from build123d import *
from OCP.BRepFilletAPI import BRepFilletAPI_MakeChamfer

# Parameters (mm, degrees)
SKETCH1_R           = 4.765
BOSS_EXTRUDE1_DEPTH = 9.5
CHAMFER1_SIZE       = 2.54
CHAMFER1_SIZE2      = 7.62
CHAMFER2_SIZE       = 7.62
CHAMFER2_SIZE2      = 2.45
CUT_EXTRUDE1_DEPTH  = 17.5
SKETCH3_W           = 9.53
SKETCH3_H           = 9.53
CUT_EXTRUDE2_DEPTH  = 17.5
SKETCH4_R           = 1.59
CUT_EXTRUDE3_DEPTH  = 17.5


with BuildPart() as part:
    # Sketch1 → Boss-Extrude1 (new, symmetric)
    with BuildSketch(Plane(origin=(0, 0, 0), x_dir=(0, 0, -1), z_dir=(1, 0, 0))):
        with BuildLine():
            Line((0, 9.765), (-22.225, 9.765))
            Line((-22.225, 9.765), (-22.225, 4.765))
            Line((-22.225, 4.765), (-9.705896356, -1.072753903))
            ThreePointArc((-9.705896356, -1.072753903), (-5.873116096, -7.801392973), (1.653013564, -9.624072483))
            Line((1.653013564, -9.624072483), (28.575, -5))
            Line((28.575, -5), (28.575, 0))
            Line((28.575, 0), (9.765, 0))
            ThreePointArc((9.765, 0), (6.904897718, 6.904897718), (0, 9.765))
        make_face()
        Circle(SKETCH1_R, mode=Mode.SUBTRACT)
    extrude(amount=BOSS_EXTRUDE1_DEPTH, both=True)

    # Chamfer1: one chamfer whose edges measure the first distance from different faces: ONE call of the kernel's chamfer builder (chamfer() names one face for all edges)
    chamfer1_edges_1 = [part.edges().sort_by_distance(p)[0] for p in [
        (9.5, 7.265, 22.225),
    ]]
    chamfer1_side_1 = [part.faces().sort_by_distance(p)[0] for p in [
        (0, 7.265, 22.225),
    ]]
    chamfer1_edges_2 = [part.edges().sort_by_distance(p)[0] for p in [
        (9.5, -2.5, -28.575),
    ]]
    chamfer1_side_2 = [part.faces().sort_by_distance(p)[0] for p in [
        (0, -2.5, -28.575),
    ]]
    chamfer1 = BRepFilletAPI_MakeChamfer(part.part.solid().wrapped)
    for e in chamfer1_edges_1:
        chamfer1.Add(CHAMFER1_SIZE, CHAMFER1_SIZE2, e.wrapped, chamfer1_side_1[0].wrapped)  # the first distance lies on this face
    for e in chamfer1_edges_2:
        chamfer1.Add(CHAMFER1_SIZE, CHAMFER1_SIZE2, e.wrapped, chamfer1_side_2[0].wrapped)  # the first distance lies on this face
    add(Compound.cast(chamfer1.Shape()), mode=Mode.REPLACE)

    # Chamfer2
    chamfer2_edges = [part.edges().sort_by_distance(p)[0] for p in [
        (-9.5, 7.265, 22.225),
        (-9.5, -2.5, -28.575),
    ]]
    chamfer2_side = [part.faces().sort_by_distance(p)[0] for p in [
        (-9.5, 9.220751812, 11.1125),
    ]]
    chamfer(chamfer2_edges, length=CHAMFER2_SIZE, length2=CHAMFER2_SIZE2, reference=chamfer2_side[0])

    # Sketch2 → Cut-Extrude1 (cut, symmetric)
    with BuildSketch(Plane(origin=(0, 0, 0), x_dir=(1, 0, 0), z_dir=(0, 1, 0))):
        with BuildLine():
            Line((5.08, 6.35), (5.08, -3.81))
            ThreePointArc((5.08, -3.81), (0, -8.89), (-5.08, -3.81))
            Line((-5.08, -3.81), (-5.08, 6.35))
            ThreePointArc((-5.08, 6.35), (0, 11.43), (5.08, 6.35))
        make_face()
    extrude(amount=CUT_EXTRUDE1_DEPTH, both=True, mode=Mode.SUBTRACT)

    # Sketch3 → Cut-Extrude2 (cut, symmetric)
    with BuildSketch(Plane(origin=(0, 0, 0), x_dir=(1, 0, 0), z_dir=(0, 1, 0))):
        with Locations((0, 23.81)):
            Rectangle(SKETCH3_W, SKETCH3_H)
        with Locations((0, -17.46)):
            Rectangle(SKETCH3_W, SKETCH3_H)
    extrude(amount=CUT_EXTRUDE2_DEPTH, both=True, mode=Mode.SUBTRACT)

    # Sketch4 → Cut-Extrude3 (cut, symmetric)
    with BuildSketch(Plane(origin=(0, 0, 0), x_dir=(0, 0, -1), z_dir=(1, 0, 0))):
        with Locations((-19.685, 7.225)):
            Circle(SKETCH4_R)
        with Locations((26.035, -2.5)):
            Circle(SKETCH4_R)
    extrude(amount=CUT_EXTRUDE3_DEPTH, both=True, mode=Mode.SUBTRACT)


solid = part.part
Part model, mm, in its own coordinate system. A direction names the side the tool comes from. Coordinates: 2 decimals unless noted, no trailing zeros. Loops run counter-clockwise (first coordinate to the right, second up) from the corner with the lowest first, then second, coordinate; pieces in that order, holes last. Notation, with made-up numbers: (23, 80) -> (62, 80) arc R17 ccw to (62, 101) -> close; hole circle Ø9 at (42.5, 88). An arc over 180 degrees is marked (long way). Use a Markdown table: item, result. Add a question column.
Item 1: Probe probe 1 along Y at (x, z) = (-6.15, 0) (3 decimals); probe 2 along X at (y, z) = (4.75, 13) (3 decimals); probe 3 along X at (y, z) = (9, -2). List the from-to ranges inside material, lowest first.
Item 2: Band-saw the part on D-D on y = -5.5. Write the cut outline in (x, z) (3 decimals).
Item 3: Flat gauge pins, fed straight in: P1, Ø1, axis at x = -0.5, z = -17, coming from the -Y side; P2, Ø5.5, axis at x = -0.5, z = -17, coming from the +Y side; P3, Ø5, axis at x = -7.5, y = -4, coming from the +Z side. Where does each tip first touch, or does it go through?
Item 4: Band-saw the part on A-A on x = 2. Write the cut outline in (y, z) (3 decimals).
Item 5: Pull direction Y, two halves, no side cores. Call faces 1 (the flat face through (-6, 7, 22.225)), 2 (the cylindrical face through (-6.145, 7.703, 18.168)), 3 (the flat face through (0, 0, -17)): +Y half, -Y half, draft (parallel to the pull), parting line (faces both ways), or undercut.
Item 6: Band-saw the part on B-B on y = 3.5. Write the cut outline in (x, z) (3 decimals).
Item 7: Which spindle directions (+Z, -Z, +X, -X, +Y, -Y) get a long thin tool onto all of the face, cutting with end or side? Do faces 4 (the flat face through (8.53, -3.2, -23.86)), 5 (the flat face through (-9.5, 4, -3)), 6 (the flat face through (-5.08, -2, -5)), 7 (the flat face through (-4.765, -3, -23)), 8 (the flat face through (0, 5, 12.695)). Say none if no direction does.
Item 8: Band-saw the part on C-C on z = -4. Write the cut outline in (x, y), plus the area to 3 significant figures.
Geometry says:
| question | item | result |
|---|---|---|
| 1 | probe 1 | -9.765 to -4.765, 4.765 to 9.765 |
| 1 | probe 2 | -9.5 to -4.765, 4.765 to 9.5 |
| 1 | probe 3 | -9.5 to -5.08, 5.08 to 9.5 |
| 2 | outline | (-9.5, -20.955) -> (-7.986, -25.664) -> (-4.765, -25.664) -> (-4.765, -19.045) -> (4.765, -19.045) -> (4.765, -25.664) -> (7.93, -25.664) -> (9.5, -20.955) -> (9.5, 8.069) -> (2.769, 8.069) arc R5.08 cw to (5.08, 3.81) -> (5.08, -6.35) arc R5.08 cw to (-5.08, -6.35) -> (-5.08, 3.81) arc R5.08 cw to (-2.769, 8.069) -> (-9.5, 8.069) -> close |
| 3 | P1 | y = -7.07 |
| 3 | P2 | y = 0 |
| 3 | P3 | z = 9.65 |
| 4 | outline | (-8.015, -11.02) -> (-6.637, -19.045) -> (0, -19.045) -> (0, -11.02) -> close; (-4.842, 8.48) -> (9.765, 8.48) -> (9.765, 12.695) -> (0.321, 12.695) -> (-1.073, 9.706) arc R9.765 ccw to start |
| 5 | face 1 | draft |
| 5 | face 2 | undercut |
| 5 | face 3 | +Y half |
| 6 | outline | (-9.5, -9.116) -> (-4.261, -9.116) arc R5.08 cw to (-5.08, -6.35) -> (-5.08, -3.233) -> (-9.5, -3.233) -> close; (-9.5, 3.233) -> (-5.08, 3.233) -> (-5.08, 3.81) arc R5.08 cw to (5.08, 3.81) -> (5.08, 3.233) -> (9.5, 3.233) -> (9.5, 14.605) -> (7.864, 19.512) -> (4.765, 19.512) -> (4.765, 12.695) -> (-4.765, 12.695) -> (-4.765, 19.512) -> (-7.922, 19.512) -> (-9.5, 14.605) -> close; (4.261, -9.116) -> (9.5, -9.116) -> (9.5, -3.233) -> (5.08, -3.233) -> (5.08, -6.35) arc R5.08 cw to start |
| 7 | face 4 | -Z, +X, +Y, -Y |
| 7 | face 5 | +Z, -Z, -X, +Y, -Y |
| 7 | face 6 | +Y, -Y |
| 7 | face 7 | -Z, +Y, -Y |
| 7 | face 8 | +Z, +Y, -Y |
| 8 | outline | (-9.5, -9.22) -> (-5.08, -9.22) -> (-5.08, -2.59) -> (-9.5, -2.59) -> close; (-9.5, 2.59) -> (-5.08, 2.59) -> (-5.08, 8.91) -> (-9.5, 8.91) -> close; (5.08, -9.22) -> (9.5, -9.22) -> (9.5, -2.59) -> (5.08, -2.59) -> close; (5.08, 2.59) -> (9.5, 2.59) -> (9.5, 8.91) -> (5.08, 8.91) -> close |
| 8 | area | 114 mm² |
